Geometry check sheet. Reference: the model listing, model coordinates, mm. Face numbers are marked on the shaded views. A direction names the side the tool comes from. Give positions to 0.01 mm unless a question says otherwise; leave off trailing zeros. Order: outer loops, then holes, each group sorted by start corner. A loop starts at its lowest first (then second) coordinate and runs counter-clockwise, first axis right, second up.
from build123d import *

# Parameters (mm, degrees)
BOSS_EXTRUDE1_DEPTH = 25
CUT_EXTRUDE1_REACH  = 60.737
SKETCH2_R           = 1.75
BOSS_EXTRUDE2_DEPTH = 10
BOSS_EXTRUDE3_START = 2
BOSS_EXTRUDE3_DEPTH = 2
SKETCH5_R           = 1.5
CUT_EXTRUDE2_DEPTH  = 117.726175299
SKETCH6_R           = 3
SKETCH6_R_2         = 1.75
CUT_EXTRUDE3_DEPTH  = 3
CUT_EXTRUDE4_START  = -3
SKETCH7_R           = 1.75
CUT_EXTRUDE4_DEPTH  = 3
SKETCH8_W           = 15
SKETCH8_H           = 14.5
BOSS_EXTRUDE4_DEPTH = 15
SKETCH9_R           = 4.75
SKETCH9_R_2         = 3.5
CUT_EXTRUDE5_DEPTH  = 3
SKETCH11_R          = 9.75
BOSS_EXTRUDE5_DEPTH = 15
CUT_EXTRUDE6_REACH  = 109.151


with BuildPart() as part:
    # Sketch1 → Boss-Extrude1 (new body)
    with BuildSketch(Plane(origin=(0, 0, 0), x_dir=(1, 0, 0), z_dir=(0, 1, 0))):
        Polygon((40, 7.5), (8, 7.5), (8, 27.5), (40, 27.5), (40, 35), (0, 35), (0, 0), (40, 0), align=None)
    extrude(amount=BOSS_EXTRUDE1_DEPTH)

    # Cut-Extrude1: up to this face of the body (flat: up to its plane)
    cut_extrude1_end = Plane(part.part.faces().sort_by_distance((20, 12.5, -35))[0])
    # Sketch2 → Cut-Extrude1 (cut, up to the picked face)
    with BuildSketch(Plane.XY, mode=Mode.PRIVATE) as cut_extrude1_sk1:
        with Locations((35.988510068, 17.617712577)):
            Circle(SKETCH2_R)
    cut_extrude1_tool1 = split(extrude(cut_extrude1_sk1.sketch, amount=-CUT_EXTRUDE1_REACH, mode=Mode.PRIVATE), bisect_by=cut_extrude1_end, keep=Keep.BOTH, mode=Mode.PRIVATE)
    # Sketch2 → Cut-Extrude1 (cut, up to the picked face)
    with BuildSketch(Plane.XY, mode=Mode.PRIVATE) as cut_extrude1_sk2:
        with Locations((12.337201721, 11.329182265)):
            Circle(SKETCH2_R)
    cut_extrude1_tool2 = split(extrude(cut_extrude1_sk2.sketch, amount=-CUT_EXTRUDE1_REACH, mode=Mode.PRIVATE), bisect_by=cut_extrude1_end, keep=Keep.BOTH, mode=Mode.PRIVATE)
    # Sketch2 → Cut-Extrude1 (cut, up to the picked face)
    with BuildSketch(Plane.XY, mode=Mode.PRIVATE) as cut_extrude1_sk3:
        Polygon((40, 25), (14.27717431, 25), (40, 20.464371811), align=None)
    cut_extrude1_tool3 = split(extrude(cut_extrude1_sk3.sketch, amount=-CUT_EXTRUDE1_REACH, mode=Mode.PRIVATE), bisect_by=cut_extrude1_end, keep=Keep.BOTH, mode=Mode.PRIVATE)
    add(cut_extrude1_tool1.solids().sort_by(Axis((35.98851, 17.617713, 0), (0, 0, -1)))[0], mode=Mode.SUBTRACT)
    add(cut_extrude1_tool2.solids().sort_by(Axis((12.337202, 11.329182, 0), (0, 0, -1)))[0], mode=Mode.SUBTRACT)
    add(cut_extrude1_tool3.solids().sort_by(Axis((31.425725, 23.488124, 0), (0, 0, -1)))[0], mode=Mode.SUBTRACT)

    # Sketch3 → Boss-Extrude2 (add)
    with BuildSketch(Plane.XZ):
        with BuildLine():
            ThreePointArc((82, 14.5), (85.535533906, 13.035533906), (87, 9.5))
            Line((87, 9.5), (87, -44.5))
            ThreePointArc((87, -44.5), (85.535533906, -48.035533906), (82, -49.5))
            Line((82, -49.5), (8, -49.5))
            ThreePointArc((8, -49.5), (4.464466094, -48.035533906), (3, -44.5))
            Line((3, -44.5), (3, -35))
            Line((3, -35), (0, -35))
            Line((0, -35), (0, -44.5))
            ThreePointArc((0, -44.5), (2.343145751, -50.156854249), (8, -52.5))
            Line((8, -52.5), (82, -52.5))
            ThreePointArc((82, -52.5), (87.656854249, -50.156854249), (90, -44.5))
            Line((90, -44.5), (90, 9.5))
            ThreePointArc((90, 9.5), (87.656854249, 15.156854249), (82, 17.5))
            Line((82, 17.5), (8, 17.5))
            ThreePointArc((8, 17.5), (2.343145751, 15.156854249), (0, 9.5))
            Line((0, 9.5), (0, 0))
            Line((0, 0), (3, 0))
            Line((3, 0), (3, 9.5))
            ThreePointArc((3, 9.5), (4.464466094, 13.035533906), (8, 14.5))
            Line((8, 14.5), (82, 14.5))
        make_face()
    extrude(amount=-BOSS_EXTRUDE2_DEPTH)

    # Sketch4 → Boss-Extrude3 (add)
    with BuildSketch(Plane.XZ.offset(BOSS_EXTRUDE3_START)):
        with BuildLine():
            Line((82, -52.5), (8, -52.5))
            ThreePointArc((8, -52.5), (2.343145751, -50.156854249), (0, -44.5))
            Line((0, -44.5), (0, 9.5))
            ThreePointArc((0, 9.5), (2.343145751, 15.156854249), (8, 17.5))
            Line((8, 17.5), (82, 17.5))
            ThreePointArc((82, 17.5), (87.656854249, 15.156854249), (90, 9.5))
            Line((90, 9.5), (90, -44.5))
            ThreePointArc((90, -44.5), (87.656854249, -50.156854249), (82, -52.5))
        make_face()
    extrude(amount=-BOSS_EXTRUDE3_DEPTH)

    # Sketch5 → Cut-Extrude2 (cut, through all)
    with BuildSketch(Plane.XY.offset(17.5)):
        with Locations((77, 5.747215229)):
            Circle(SKETCH5_R)
    extrude(amount=-CUT_EXTRUDE2_DEPTH, mode=Mode.SUBTRACT)

    # Sketch6 → Cut-Extrude3 (cut)
    # profile 1 of 2: a face of its own
    with BuildSketch(Plane.XY):
        with Locations((12.337201721, 11.329182265)):
            Circle(SKETCH6_R)
        with Locations((12.337201721, 11.329182265)):
            Circle(SKETCH6_R_2, mode=Mode.SUBTRACT)
    # profile 2 of 2: a face of its own
    with BuildSketch(Plane.XY):
        with Locations((35.988510068, 17.617712577)):
            Circle(SKETCH6_R)
        with Locations((35.988510068, 17.617712577)):
            Circle(SKETCH6_R_2, mode=Mode.SUBTRACT)
    extrude(amount=-CUT_EXTRUDE3_DEPTH, mode=Mode.SUBTRACT)

    # Sketch7 → Cut-Extrude4 (cut)
    # profile 1 of 2: a face of its own
    with BuildSketch(Plane(origin=(0, 0, -35), x_dir=(-1, 0, 0), z_dir=(0, 0, -1)).offset(CUT_EXTRUDE4_START)):
        Polygon((-37.576223308, 14.867712577), (-34.400796828, 14.867712577), (-32.813083587, 17.617712577), (-34.400796828, 20.367712577), (-37.576223308, 20.367712577), (-39.163936548, 17.617712577), align=None)
        with Locations((-35.988510068, 17.617712577)):
            Circle(SKETCH7_R, mode=Mode.SUBTRACT)
    # profile 2 of 2: a face of its own
    with BuildSketch(Plane(origin=(0, 0, -35), x_dir=(-1, 0, 0), z_dir=(0, 0, -1)).offset(CUT_EXTRUDE4_START)):
        Polygon((-13.924914961, 8.579182265), (-10.749488481, 8.579182265), (-9.16177524, 11.329182265), (-10.749488481, 14.079182265), (-13.924914961, 14.079182265), (-15.512628201, 11.329182265), align=None)
        with Locations((-12.337201721, 11.329182265)):
            Circle(SKETCH7_R, mode=Mode.SUBTRACT)
    extrude(amount=CUT_EXTRUDE4_DEPTH, mode=Mode.SUBTRACT)

    # Sketch8 → Boss-Extrude4 (add)
    with BuildSketch(Plane(origin=(0, 0, 0), x_dir=(1, 0, 0), z_dir=(0, 1, 0))):
        with Locations((24, -7.25)):
            Rectangle(SKETCH8_W, SKETCH8_H)
        with Locations((24, 42.25)):
            Rectangle(SKETCH8_W, SKETCH8_H)
    extrude(amount=BOSS_EXTRUDE4_DEPTH)

    # Sketch9 → Cut-Extrude5 (cut)
    # profile 1 of 2: a face of its own
    with BuildSketch(Plane(origin=(0, 15, 0), x_dir=(1, 0, 0), z_dir=(0, 1, 0))):
        with Locations(Location((24, 42.25, 0), (0, 0, 270))):
            Circle(SKETCH9_R)
        with Locations(Location((24, 42.25, 0), (0, 0, 270))):
            Circle(SKETCH9_R_2, mode=Mode.SUBTRACT)
    # profile 2 of 2: a face of its own
    with BuildSketch(Plane(origin=(0, 15, 0), x_dir=(1, 0, 0), z_dir=(0, 1, 0))):
        with Locations(Location((24, -7.25, 0), (0, 0, 270))):
            Circle(SKETCH9_R)
        with Locations(Location((24, -7.25, 0), (0, 0, 270))):
            Circle(SKETCH9_R_2, mode=Mode.SUBTRACT)
    extrude(amount=-CUT_EXTRUDE5_DEPTH, mode=Mode.SUBTRACT)

    # Sketch11 → Boss-Extrude5 (add)
    with BuildSketch(Plane(origin=(0, 0, 0), x_dir=(1, 0, 0), z_dir=(0, 1, 0))):
        with Locations(Location((67, 30, 0), (0, 0, 90))):
            Circle(SKETCH11_R)
        with Locations(Location((67, 5, 0), (0, 0, 90))):
            Circle(SKETCH11_R)
    extrude(amount=BOSS_EXTRUDE5_DEPTH)

    # Sketch12 → Cut-Extrude6 (cut, up to next)
    with BuildSketch(Plane.ZY, mode=Mode.PRIVATE) as cut_extrude6_sk1:
        with BuildLine():
            Line((-20, 7.759198983), (-20, 2.5))
            ThreePointArc((-20, 2.5), (-17.5, 0), (-15, 2.5))
            Line((-15, 2.5), (-15, 7.759198983))
            ThreePointArc((-15, 7.759198983), (-17.5, 20.259198983), (-20, 7.759198983))
        make_face()
    cut_extrude6_tool1 = extrude(cut_extrude6_sk1.sketch, amount=-CUT_EXTRUDE6_REACH, mode=Mode.PRIVATE) & part.part
    add(cut_extrude6_tool1.solids().sort_by_distance((0, 11.74048, -17.5))[0], mode=Mode.SUBTRACT)


solid = part.part
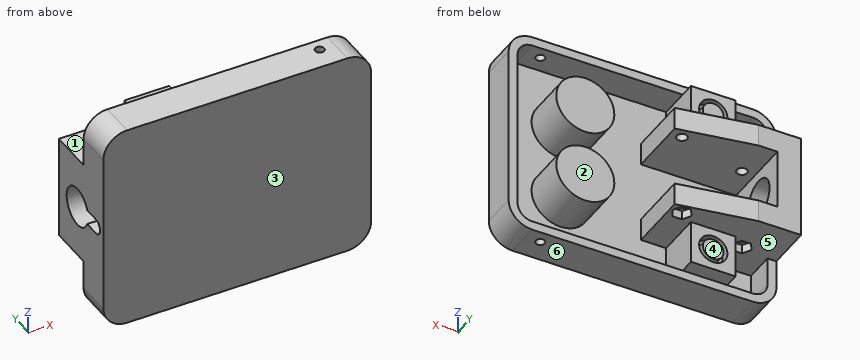
Item 1: Sectioned sample at C-C (z = 7.25). Enter the section's corners in (x, y), and give its area (4 significant figures).
Reported:
outline: (0, -2) - (90, -2) - (90, 10) - (87, 10) - (87, 0) - (31.5, 0) - (31.5, 15) - (28.75, 15) - (28.75, 12) - (27.5, 12) - (27.5, 15) - (20.5, 15) - (20.5, 12) - (19.25, 12) - (19.25, 15) - (16.5, 15) - (16.5, 0) - (3, 0) - (3, 10) - (0, 10) - close
area: 457.5 mm2
Item 2: Draft check along Z on the marked faces 4, 5 and 6. Enter one of: released by +Z, released by -Z, zero draft, split by the parting line, or undercut.
Reported:
face 4: zero draft
face 5: undercut
face 6: released by -Z
Item 3: Sectioned sample at B-B (z = -30). Enter the section's corners in (x, y).
Reported:
outline: (0, -2) - (90, -2) - (90, 10) - (87, 10) - (87, 0) - (76.75, 0) - (76.75, 15) - (57.25, 15) - (57.25, 0) - (40, 0) - (40, 20.46) - (14.28, 25) - (0, 25) - close; hole circle Ø3.5 at (12.34, 11.33); hole circle Ø3.5 at (35.99, 17.62)
Item 4: Sectioned sample at A-A (x = 7). Enter the section's corners in (y, z), and give its area (3 significant figures).
Reported:
outline: (-2, -52.44) - (10, -52.44) - (10, -49.4) - (0, -49.4) - (0, -35) - (25, -35) - (25, 0) - (0, 0) - (0, 14.4) - (10, 14.4) - (10, 17.44) - (-2, 17.44) - close; hole (2.5, -20) - (7.76, -20) arc R6.5 ccw (long way) to (7.76, -15) - (2.5, -15) arc R2.5 ccw to start
area: 908 mm2
Item 5: Set-up check for the marked faces 1, 2 and 3: record each of +Z, -Z, +X, -X, +Y, -Y from which the full face is reachable in a straight line by a thin tool's end or side.
Reported:
face 1: +Y
face 2: +Z, -Z, +X, +Y
face 3: +Z, -Z, +X, -X, -Y
Item 6: Gauge pin test, flat ends, axial feed: pin 1 (1 mm diameter, centred on x = 25, z = 8, fed in from +Y); pin 2 (2 mm diameter, centred on x = 60.5, y = 15.5, fed in from -Z); pin 3 (3 mm diameter, centred on x = 35.99, y = 17.62, fed in from +Z); pin 4 (3.5 mm diameter, centred on x = 36.5, z = -33, fed in from +Y). Record the tip position at first contact, or that the pin passes through.
Reported:
pin 1: stops at y = 15
pin 2: stops at z = -37.96
pin 3: passes through
pin 4: stops at y = 21.39
Item 7: Scan lines: L1, parallel to Z at x = 39, y = 6; L2, parallel to Z at x = 11, y = 9.5; L3, parallel to Z at x = 51.5, y = 9.25. Record each from-to range of solid material in increasing order.
Reported:
L1: z = -52.5 to -49.5, -35 to -27.5, -7.5 to 0, 14.5 to 17.5
L2: z = -52.5 to -49.5, -32 to -27.5, -7.5 to -3, 14.5 to 17.5
L3: z = -52.5 to -49.5, 14.5 to 17.5
